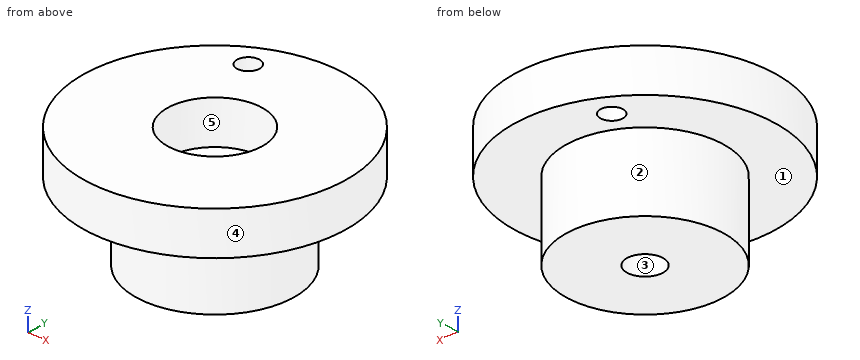
```python
from build123d import *

# Parameters (mm, degrees)
SKETCH_1_R          = 29
SKETCH_1_R_2        = 10.5
EXTRUDE_1_DEPTH     = 9.5
SKETCH_2_R          = 17.5
SKETCH_2_R_2        = 4
EXTRUDE_2_DEPTH     = 17
SKETCH_3_R          = 2.5
CUT_EXTRUDE_1_DEPTH = 17


with BuildPart() as part:
    # Эскиз1 → Бобышка-Вытянуть1 (new body)
    with BuildSketch(Plane.XY):
        Circle(SKETCH_1_R)
        Circle(SKETCH_1_R_2, mode=Mode.SUBTRACT)
    extrude(amount=EXTRUDE_1_DEPTH)

    # Эскиз2 → Бобышка-Вытянуть2 (add)
    with BuildSketch(Plane(origin=(0, 0, 0), x_dir=(-1, 0, 0), z_dir=(0, 0, -1))):
        Circle(SKETCH_2_R)
        Circle(SKETCH_2_R_2, mode=Mode.SUBTRACT)
    extrude(amount=EXTRUDE_2_DEPTH)

    # Эскиз3 → Вырез-Вытянуть1 (cut)
    with BuildSketch(Plane.XY.offset(9.5)):
        with Locations((-10.871713138, 20.268346096)):
            Circle(SKETCH_3_R)
    extrude(amount=-CUT_EXTRUDE_1_DEPTH, mode=Mode.SUBTRACT)


solid = part.part
```
Can you work these out from the model? Positions are in its coordinate system, mm. Face numbers are marked on the shaded views. A direction names the side the tool comes from. Coordinates: 2 decimals unless noted, no trailing zeros. Write each loop counter-clockwise with the first axis right and the second up, starting at its lowest first coordinate (ties: lowest second). Pieces come first, ordered by that corner, then holes. Notation, with made-up numbers: M 9.25,-19.5 L 58.25,-19.5 A22 cw 58.25,16.5 Z; hole C 46,-11 d11. An arc over 180 degrees is marked long. Write item = value, one per line. Start each with the question number.
Q1. If we section it at C-C, the plane z = -10.25: Write out the boundary of the cut face in (x, y), then the cut area to 3 significant figures.
Q2. I'm going to push flat-ended pins straight in: pin 1 (1.5 mm diameter, centred on x = -1, y = -1.5, fed in from +Z); pin 2 (8 mm diameter, centred on x = -13, y = -22, fed in from -Z); pin 3 (6.5 mm diameter, centred on x = -1.5, y = 3.5, fed in from +Z); pin 4 (1.5 mm diameter, centred on x = -10.5, z = -3.5, fed in from -Y). Where does each tip first touch, or does it pass through?
Q3. If I drill on L1, parallel to Y at x = 0, z = -4.5; L2, parallel to Y at x = -12.5, z = 3.5; L3, parallel to Z at x = 21.5, y = 18, over which ranges is the centre line in solid material (lowest first)? Write a range as [from, to].
Q4. Thinking about a two-plate mould opening in X: for the marked faces 1, 2 and 3, which applies, released by +X, released by -X, zero draft, split by the parting line, or undercut?
Q5. On a 3-axis mill with a long thin cutter (end or side, diameter ignored), from which of +Z, -Z, +X, -X, +Y, -Y can I reach the whole of each face in a straight line? I mean the marked faces 4 and 5. Say none if no direction works.
Q6. If we section it at A-A, the plane x = 0: Write out the boundary of the cut face in (y, z), then the cut area to 4 significant figures.
Q7. If we section it at D-D, the plane x = -12.5: Write out the boundary of the cut face in (y, z).
Check sheet entries:
q1.outline = C 0,0 d35; hole C 0,0 d8
q1.area = 912 mm²
q2.pin_1 = through
q2.pin_2 = 0
q2.pin_3 = 0
q2.pin_4 = -14.53
q3.L1 = [-17.5, -4], [4, 17.5]
q3.L2 = [-26.17, 18.37], [22.17, 26.17]
q3.L3 = [0, 9.5]
q4.face_1 = zero draft
q4.face_2 = split by the parting line
q4.face_3 = undercut
q5.face_4 = +Z, -Z
q5.face_5 = +Z
q6.outline = M -29,0 L -17.5,0 L -17.5,-17 L -4,-17 L -4,0 L -10.5,0 L -10.5,9.5 L -29,9.5 Z; M 4,-17 L 17.5,-17 L 17.5,0 L 29,0 L 29,9.5 L 10.5,9.5 L 10.5,0 L 4,0 Z
q6.area = 810.5 mm²
q7.outline = M -26.17,0 L -12.25,0 L -12.25,-17 L 12.25,-17 L 12.25,0 L 18.37,0 L 18.37,9.5 L -26.17,9.5 Z; M 22.17,0 L 26.17,0 L 26.17,9.5 L 22.17,9.5 Z
